Source: three-view drawing plus pictorial views. Frame: mm from the lowest corner of the part. Give positions to 0.01 mm unless a question says otherwise; leave off trailing zeros. Write each loop counter-clockwise with the first axis right and the second up, starting at its lowest first coordinate (ties: lowest second). Pieces come first, ordered by that corner, then holes. Notation, with made-up numbers: M 75,55 L 134,55 A28 ccw 134,83 Z; hole C -20.75,2 d6. An arc over 180 degrees is marked long. One line per question, with ' | ' between items.
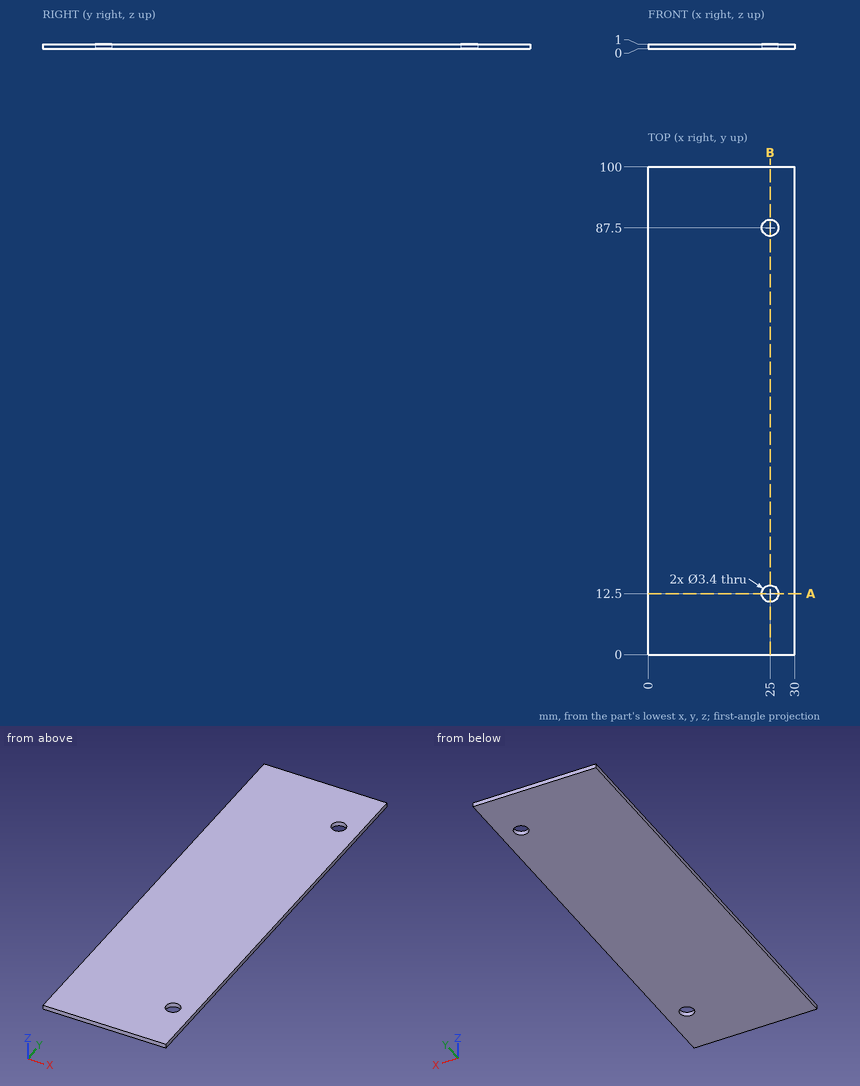
(1) Cut plane B-B, the plane x = 25. Return loops of the section in (y, z), then the cut area to 3 significant figures.
Working result:
outline: M 0,0 L 10.8,0 L 10.8,1 L 0,1 Z; M 14.2,0 L 85.8,0 L 85.8,1 L 14.2,1 Z; M 89.2,0 L 100,0 L 100,1 L 89.2,1 Z | area: 93.2 mm^2
(2) First-contact query: P1, Ø3, axis at x = 25, y = 12.5, coming from the +Z side. Flat tip, straight axial feed; report the tip coordinate or a pass-through.
Working result:
P1: passes through
(3) Cut plane A-A, the plane y = 12.5. Return loops of the section in (x, z), then the cut area to 3 significant figures.
Working result:
outline: M 0,0 L 23.3,0 L 23.3,1 L 0,1 Z; M 26.7,0 L 30,0 L 30,1 L 26.7,1 Z | area: 26.6 mm^2
(4) Material intervals for L1, parallel to Y at x = 25, z = 0.55; L2, parallel to X at y = 12.5, z = 0.3, sorted ascending. Write a range as [from, to].
Working result:
L1: y = [0, 10.8], [14.2, 85.8], [89.2, 100] | L2: x = [0, 23.3], [26.7, 30]
